```python
from build123d import *

# Parameters (mm, degrees)
SKETCH1_R          = 2
EXTRUDE1_DEPTH     = 14
SKETCH6_R          = 4
EXTRUDE2_DEPTH     = 2.3
CUT_EXTRUDE1_DEPTH = 1.875


with BuildPart() as part:
    # Sketch1 → Extrude1 (new body)
    with BuildSketch(Plane.XY):
        Circle(SKETCH1_R)
    extrude(amount=-EXTRUDE1_DEPTH)

    # Sketch6 → Extrude2 (add)
    with BuildSketch(Plane(origin=(0, 0, -14), x_dir=(-1, 0, 0), z_dir=(0, 0, -1))):
        Circle(SKETCH6_R)
    extrude(amount=-EXTRUDE2_DEPTH)

    # Sketch10 → Cut-Revolve2 (revolve, cut)
    with BuildSketch(Plane(origin=(0, 0, 0), x_dir=(0, 0, -1), z_dir=(1, 0, 0)), mode=Mode.PRIVATE) as cut_revolve2_sk:
        Polygon((13.7, -4), (11.7, -2), (11.7, -4), align=None)
    revolve(cut_revolve2_sk.sketch.rotate(Axis((0, 0, 0), (0, 0, -1)), 90), axis=Axis((0, 0, 0), (0, 0, -1)), mode=Mode.SUBTRACT)

    # Sketch7 → Cut-Extrude1 (cut)
    with BuildSketch(Plane.XY.offset(-14)):
        Polygon((0, 1.443375673), (-1.25, 0.721687836), (-1.25, -0.721687836), (0, -1.443375673), (1.25, -0.721687836), (1.25, 0.721687836), align=None)
    extrude(amount=CUT_EXTRUDE1_DEPTH, mode=Mode.SUBTRACT)


solid = part.part
```
Design review of the part built by this model. Coordinates are the model's own, in mm. A direction names the side the tool comes from. Round coordinates to 2 decimals unless told otherwise and drop trailing zeros. Order: outer loops, then holes, each group sorted by start corner. A loop starts at its lowest first (then second) coordinate and runs counter-clockwise, first axis right, second up. Notation, with made-up numbers: M 67,27.5 L 107,27.5 A20 cw 107,54.5 Z; hole C 45,30.25 d3. An arc over 180 degrees is marked long. Put each result on its own line as item: value.
Q1. Insertion check: pin 1 Ø1.5 at (y, z) = (1, -6.5) entering from -X; pin 2 Ø0.7 at (y, z) = (0.5, -13) entering from +X; pin 3 Ø4 at (y, z) = (-2, -12.5) entering from -X. Each pin has a flat end and moves straight along its axis. Give the tip position at first contact, or say it passes through.
Reported:
pin 1: x = -1.98
pin 2: x = 3.62
pin 3: x = -3.98
Q2. Machinability: for faces 4 (the face through (0, 0, 0)), 5 (the face through (-0.616, 1.088, -13.076)), which of the approach directions +Z, -Z, +X, -X, +Y, -Y give a long, thin tool a straight path to every point of the face, cutting with its end or side? Answer none if there is none.
Reported:
face 4: +Z, +X, -X, +Y, -Y
face 5: -Z
Q3. Draft analysis for pull direction X (two halves, no side actions). For faces 1 (the face through (-2, 0, -14)), 2 (the face through (0, -2, -6)), 3 (the face through (0, 0, -12.125)), state which applies: released by +X, released by -X, zero draft, split by the parting line, or undercut.
Reported:
face 1: zero draft
face 2: split by the parting line
face 3: undercut
Q4. Consider section B-B (z = -11). State the section outline as (x, y) points, and give its area (3 significant figures).
Reported:
outline: C 0,0 d4
area: 12.6 mm²
Q5. To check wall thickness, follow line 1 (X direction, y = 0, z = -2.5); line 2 (Z direction, x = 0.5, y = 0.5) (3 decimals); line 3 (Z direction, x = 1.5, y = -1.5). State the ranges of each line that lie inside material, in increasing order.
Reported:
line 1: -2 to 2
line 2: -12.125 to 0
line 3: -14 to -11.82
Q6. Consider section A-A (y = 0). State the section outline as (x, z) points (3 decimals), and give its area (3 significant figures).
Reported:
outline: M -4,-14 L -1.25,-14 L -1.25,-12.125 L 1.25,-12.125 L 1.25,-14 L 4,-14 L 4,-13.7 L 2,-11.7 L 2,0 L -2,0 L -2,-11.7 L -4,-13.7 Z
area: 56.5 mm²
